Could you check a few things on this model? Use its own coordinates, in mm. Give positions to 0.01 mm unless a question says otherwise; leave off trailing zeros. Loops run counter-clockwise (first coordinate to the right, second up) from the corner with the lowest first, then second, coordinate; pieces in that order, holes last. Notation, with made-up numbers: (64, -3) -> (76, -3) arc R18 ccw to (76, 25) -> close; hole circle Ø8 at (71, 49.25). An arc over 180 degrees is marked (long way). Put each result on its own line as item: value.
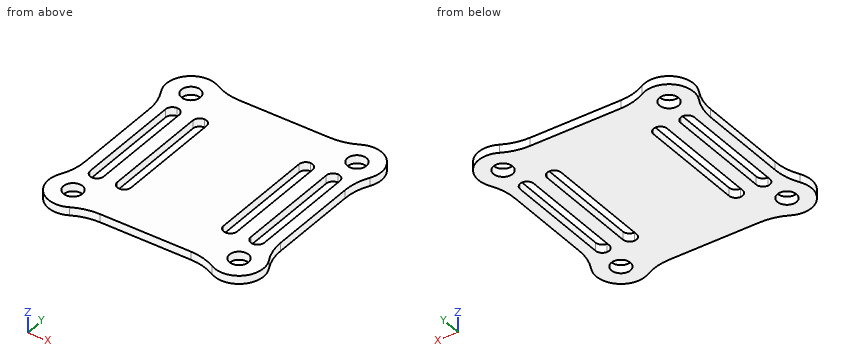
```python
from build123d import *

# Parameters (mm, degrees)
F0_W     = 36
F0_H     = 36
F1_DEPTH = 1.5
F2_R     = 4.5
F3_DEPTH = 1.5
F4_R     = 1.75
F5_DEPTH = 1.501
F7_DEPTH = 1.501
F8_R     = 10


with BuildPart() as f1:
    # F0 (on Top) → F1 (new body)
    with BuildSketch(Plane.XY):
        Rectangle(F0_W, F0_H)
    extrude(amount=F1_DEPTH)

    # F2 (on Top) → F3 (join)
    with BuildSketch(Plane.XY):
        with Locations((-15.25, 15.25)):
            Circle(F2_R)
        with Locations((15.25, 15.25)):
            Circle(F2_R)
        with Locations((-15.25, -15.25)):
            Circle(F2_R)
        with Locations((15.25, -15.25)):
            Circle(F2_R)
    extrude(amount=F3_DEPTH)

    # F4 (on face) → F5 (cut, through all)
    with BuildSketch(Plane.XY.offset(1.5)):
        with Locations((-15.25, -15.25)):
            Circle(F4_R)
        with Locations((15.25, -15.25)):
            Circle(F4_R)
        with Locations((-15.25, 15.25)):
            Circle(F4_R)
        with Locations((15.25, 15.25)):
            Circle(F4_R)
    extrude(amount=-F5_DEPTH, mode=Mode.SUBTRACT)

    # F6 (on face) → F7 (cut, through all)
    with BuildSketch(Plane.XY.offset(1.5)):
        with BuildLine():
            ThreePointArc((-9.75, 11), (-10.6338834765, 10.6338834765), (-11, 9.75))
            Line((-11, 9.75), (-11, -9.75))
            ThreePointArc((-11, -9.75), (-10.6338834765, -10.6338834765), (-9.75, -11))
            ThreePointArc((-9.75, -11), (-8.8661165235, -10.6338834765), (-8.5, -9.75))
            Line((-8.5, -9.75), (-8.5, 9.75))
            ThreePointArc((-8.5, 9.75), (-8.8661165235, 10.6338834765), (-9.75, 11))
        make_face()
        with BuildLine():
            ThreePointArc((-14.75, 11), (-15.6338834765, 10.6338834765), (-16, 9.75))
            Line((-16, 9.75), (-16, -9.75))
            ThreePointArc((-16, -9.75), (-15.6338834765, -10.6338834765), (-14.75, -11))
            ThreePointArc((-14.75, -11), (-13.8661165235, -10.6338834765), (-13.5, -9.75))
            Line((-13.5, -9.75), (-13.5, 9.75))
            ThreePointArc((-13.5, 9.75), (-13.8661165235, 10.6338834765), (-14.75, 11))
        make_face()
        with BuildLine():
            ThreePointArc((9.75, 11), (8.8661165235, 10.6338834765), (8.5, 9.75))
            Line((8.5, 9.75), (8.5, -9.75))
            ThreePointArc((8.5, -9.75), (8.8661165235, -10.6338834765), (9.75, -11))
            ThreePointArc((9.75, -11), (10.6338834765, -10.6338834765), (11, -9.75))
            Line((11, -9.75), (11, 9.75))
            ThreePointArc((11, 9.75), (10.6338834765, 10.6338834765), (9.75, 11))
        make_face()
        with BuildLine():
            Line((16, -9.75), (16, 9.75))
            ThreePointArc((16, 9.75), (15.6338834765, 10.6338834765), (14.75, 11))
            ThreePointArc((14.75, 11), (13.8661165235, 10.6338834765), (13.5, 9.75))
            Line((13.5, 9.75), (13.5, -9.75))
            ThreePointArc((13.5, -9.75), (13.8661165235, -10.6338834765), (14.75, -11))
            ThreePointArc((14.75, -11), (15.6338834765, -10.6338834765), (16, -9.75))
        make_face()
    extrude(amount=-F7_DEPTH, mode=Mode.SUBTRACT)

    # F8
    f8_edges = [f1.edges().sort_by_distance(p)[0] for p in [
        (-18, 11.688048, 0.75),
        (-11.688048, 18, 0.75),
        (11.688048, 18, 0.75),
        (18, 11.688048, 0.75),
        (18, -11.688048, 0.75),
        (11.688048, -18, 0.75),
        (-11.688048, -18, 0.75),
        (-18, -11.688048, 0.75),
    ]]
    fillet(f8_edges, radius=F8_R)


solid = f1.part
```
1. I'm going to push a flat-ended pin straight in: pin 1 (0.8 mm diameter, centred on y = 3.5, z = 1, fed in from -X). Where does the tip first touch, or does it pass through?
Recorded:
pin 1: stops at x = -18
2. If we section it at B-B (y = 7): List the corners of the cut face in (x, z) for me, then the cut area to 3 significant figures.
Recorded:
outline: (-18, 0) -> (-16, 0) -> (-16, 1.5) -> (-18, 1.5) -> close; (-13.5, 0) -> (-11, 0) -> (-11, 1.5) -> (-13.5, 1.5) -> close; (-8.5, 0) -> (8.5, 0) -> (8.5, 1.5) -> (-8.5, 1.5) -> close; (11, 0) -> (13.5, 0) -> (13.5, 1.5) -> (11, 1.5) -> close; (16, 0) -> (18, 0) -> (18, 1.5) -> (16, 1.5) -> close
area: 39.0 mm^2
3. I need wall thicknesses on line 1 (X direction, y = -6, z = 1.15); line 2 (X direction, y = -14, z = 0.2); line 3 (Y direction, x = 15.25, z = 1.05). Which ranges of each line are inside material? Lowest first, please.
Recorded:
line 1: x = -18 to -16, -13.5 to -11, -8.5 to 8.5, 11 to 13.5, 16 to 18
line 2: x = -19.57 to -16.47, -14.03 to 14.03, 16.47 to 19.57
line 3: y = -19.75 to -17, -13.5 to -10.9, 10.9 to 13.5, 17 to 19.75
4. If we section it at D-D (z = 0.8): Count the separate pieces of the cut face and the enclosed holes in it, then the cut area to 3 significant figures.
Recorded:
separate pieces: 1
enclosed holes: 8
area: 1,120 mm^2
5. If we section it at C-C (x = -15.5): List the corners of the cut face in (y, z) for me, then the cut area to 3 significant figures.
Recorded:
outline: (-19.74, 0) -> (-16.98, 0) -> (-16.98, 1.5) -> (-19.74, 1.5) -> close; (-13.52, 0) -> (-10.75, 0) -> (-10.75, 1.5) -> (-13.52, 1.5) -> close; (10.75, 0) -> (13.52, 0) -> (13.52, 1.5) -> (10.75, 1.5) -> close; (16.98, 0) -> (19.74, 0) -> (19.74, 1.5) -> (16.98, 1.5) -> close
area: 16.6 mm^2
6. If we section it at A-A (y = 15.25): List the corners of the cut face in (x, z) for me.
Recorded:
outline: (-19.75, 0) -> (-17, 0) -> (-17, 1.5) -> (-19.75, 1.5) -> close; (-13.5, 0) -> (13.5, 0) -> (13.5, 1.5) -> (-13.5, 1.5) -> close; (17, 0) -> (19.75, 0) -> (19.75, 1.5) -> (17, 1.5) -> close
